Verification items for the finished model (mm, model axes). Face numbers are marked on the shaded views. A direction names the side the tool comes from. Round coordinates to 2 decimals unless told otherwise and drop trailing zeros. Loops run counter-clockwise (first coordinate to the right, second up) from the corner with the lowest first, then second, coordinate; pieces in that order, holes last. Notation, with made-up numbers: (-33, 42.5) -> (-25, 42.5) arc R19 ccw to (-25, 54.5) -> close; hole circle Ø2 at (-9.5, -22.5). An arc over 180 degrees is marked (long way). Write item = value, one per line. Start each with the question number.
```python
from build123d import *

# Parameters (mm, degrees)
F1_DEPTH = 1.27
F2_W     = 3.175
F2_H     = 3.175
F3_DEPTH = 25.4


with BuildPart() as f1:
    # F0 (on Front) → F1 (new body)
    with BuildSketch(Plane.XZ):
        with BuildLine():
            Line((2.9464038958, -0.7894865445), (0, 0))
            Line((0, 0), (3.0794409887, 0.8251337261))
            Line((3.0794409887, 0.8251337261), (2.99397894, 1.1440824339))
            Line((2.99397894, 1.1440824339), (3.3486255796, 1.4393611732))
            ThreePointArc((3.3486255796, 1.4393611732), (3.1918481536, 1.8075915845), (2.9973088366, 2.1573447134))
            Line((2.9973088366, 2.1573447134), (2.6208310146, 2.0564677851))
            Line((2.6208310146, 2.0564677851), (2.3873443555, 2.2899544442))
            Line((2.3873443555, 2.2899544442), (2.1538576963, 2.5234411034))
            Line((2.1538576963, 2.5234411034), (2.3133513259, 2.9564833127))
            ThreePointArc((2.3133513259, 2.9564833127), (1.9934628866, 3.1969914902), (1.6501103316, 3.4026169264))
            Line((1.6501103316, 3.4026169264), (1.374509438, 3.1270160328))
            Line((1.374509438, 3.1270160328), (1.0555607301, 3.2124780815))
            Line((1.0555607301, 3.2124780815), (0.7366120223, 3.2979401302))
            Line((0.7366120223, 3.2979401302), (0.6582164526, 3.7527124992))
            ThreePointArc((0.6582164526, 3.7527124992), (0.2609308491, 3.8010544711), (-0.1392339042, 3.807455045))
            Line((-0.1392339042, 3.807455045), (-0.2401108325, 3.430977223))
            Line((-0.2401108325, 3.430977223), (-0.5590595404, 3.3455151743))
            Line((-0.5590595404, 3.3455151743), (-0.8780082482, 3.2600531257))
            Line((-0.8780082482, 3.2600531257), (-1.1732869876, 3.6146997653))
            ThreePointArc((-1.1732869876, 3.6146997653), (-1.5415173988, 3.4579223392), (-1.8912705277, 3.2633830223))
            Line((-1.8912705277, 3.2633830223), (-1.7903935994, 2.8869052003))
            Line((-1.7903935994, 2.8869052003), (-2.0238802585, 2.6534185411))
            Line((-2.0238802585, 2.6534185411), (-2.2573669177, 2.419931882))
            Line((-2.2573669177, 2.419931882), (-2.690409127, 2.5794255116))
            ThreePointArc((-2.690409127, 2.5794255116), (-2.9309173045, 2.2595370723), (-3.1365427408, 1.9161845173))
            Line((-3.1365427408, 1.9161845173), (-2.8609418471, 1.6405836237))
            Line((-2.8609418471, 1.6405836237), (-2.9464038958, 1.3216349158))
            Line((-2.9464038958, 1.3216349158), (-3.0318659445, 1.002686208))
            Line((-3.0318659445, 1.002686208), (-3.4866383135, 0.9242906383))
            ThreePointArc((-3.4866383135, 0.9242906383), (-3.5349802854, 0.5270050347), (-3.5413808594, 0.1268402815))
            Line((-3.5413808594, 0.1268402815), (-3.1649030374, 0.0259633531))
            Line((-3.1649030374, 0.0259633531), (-3.0794409887, -0.2929853547))
            Line((-3.0794409887, -0.2929853547), (-2.99397894, -0.6119340625))
            Line((-2.99397894, -0.6119340625), (-3.3486255796, -0.9072128019))
            ThreePointArc((-3.3486255796, -0.9072128019), (-3.1918481536, -1.2754432131), (-2.9973088366, -1.6251963421))
            Line((-2.9973088366, -1.6251963421), (-2.6208310146, -1.5243194137))
            Line((-2.6208310146, -1.5243194137), (-2.3873443555, -1.7578060728))
            Line((-2.3873443555, -1.7578060728), (-2.1538576963, -1.991292732))
            Line((-2.1538576963, -1.991292732), (-2.3133513259, -2.4243349413))
            ThreePointArc((-2.3133513259, -2.4243349413), (-1.9934628866, -2.6648431188), (-1.6501103316, -2.8704685551))
            Line((-1.6501103316, -2.8704685551), (-1.374509438, -2.5948676615))
            Line((-1.374509438, -2.5948676615), (-1.0555607301, -2.6803297101))
            Line((-1.0555607301, -2.6803297101), (-0.7366120223, -2.7657917588))
            Line((-0.7366120223, -2.7657917588), (-0.6582164526, -3.2205641278))
            ThreePointArc((-0.6582164526, -3.2205641278), (-0.2609308491, -3.2689060997), (0.1392339042, -3.2753066737))
            Line((0.1392339042, -3.2753066737), (0.2401108325, -2.8988288517))
            Line((0.2401108325, -2.8988288517), (0.5590595404, -2.813366803))
            Line((0.5590595404, -2.813366803), (0.8780082482, -2.7279047543))
            Line((0.8780082482, -2.7279047543), (1.1732869876, -3.0825513939))
            ThreePointArc((1.1732869876, -3.0825513939), (1.5415173988, -2.9257739679), (1.8912705277, -2.7312346509))
            Line((1.8912705277, -2.7312346509), (1.7903935994, -2.3547568289))
            Line((1.7903935994, -2.3547568289), (2.0238802585, -2.1212701698))
            Line((2.0238802585, -2.1212701698), (2.2573669177, -1.8877835106))
            Line((2.2573669177, -1.8877835106), (2.690409127, -2.0472771403))
            ThreePointArc((2.690409127, -2.0472771403), (2.9309173045, -1.7273887009), (3.1365427408, -1.3840361459))
            Line((3.1365427408, -1.3840361459), (2.8609418471, -1.1084352523))
            Line((2.8609418471, -1.1084352523), (2.9464038958, -0.7894865445))
        make_face()
        with BuildLine():
            ThreePointArc((3.4866383135, -0.392142267), (3.4939098929, -0.3492466485), (3.5006911676, -0.3062707917))
            Line((3.5006911676, -0.3062707917), (0, 0))
            Line((0, 0), (2.9464038958, -0.7894865445))
            Line((2.9464038958, -0.7894865445), (3.0318659445, -0.4705378366))
            Line((3.0318659445, -0.4705378366), (3.4866383135, -0.392142267))
        make_face()
        with BuildLine():
            ThreePointArc((3.5439258143, 0.2660741857), (3.5438624188, 0.2880530324), (3.5436722344, 0.3100311478))
            Line((3.5436722344, 0.3100311478), (0, 0))
            Line((0, 0), (3.5006911676, -0.3062707917))
            ThreePointArc((3.5006911676, -0.3062707917), (3.5331017773, -0.0209136223), (3.5439258143, 0.2660741857))
        make_face()
        with BuildLine():
            Line((0, 0), (3.5436722344, 0.3100311478))
            ThreePointArc((3.5436722344, 0.3100311478), (3.5428244693, 0.3576767837), (3.5413808594, 0.4053080898))
            Line((3.5413808594, 0.4053080898), (3.1649030374, 0.5061850182))
            Line((3.1649030374, 0.5061850182), (3.0794409887, 0.8251337261))
            Line((3.0794409887, 0.8251337261), (0, 0))
        make_face()
    extrude(amount=F1_DEPTH)

    # F2 (on face) → F3 (cut)
    with BuildSketch(Plane.XZ.offset(1.27)):
        with Locations((0, 0.2660741857)):
            Rectangle(F2_W, F2_H)
    extrude(amount=-F3_DEPTH, mode=Mode.SUBTRACT)


solid = f1.part
```
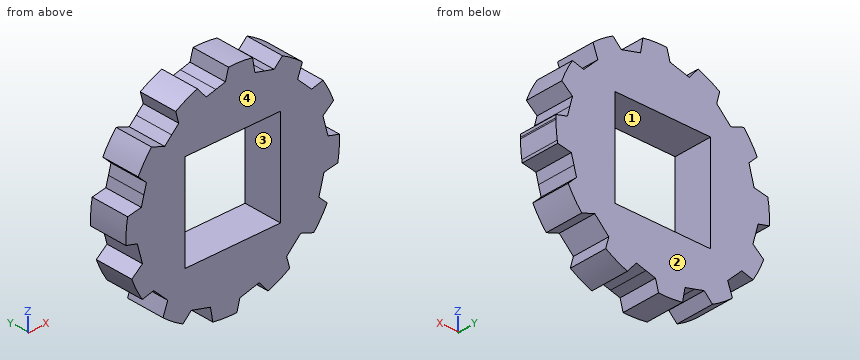
(1) Draft check along Z on the marked faces 3 and 4. Enter one of: +Z half, -Z half, draft (parallel to the pull), parting line (faces both ways), or undercut.
(2) Section check C-C on x = -2.5. Enter the section's corners in (y, z), then the cut area to 3 significant figures.
(3) Section check A-A on z = 1.75. Enter the section's corners in (x, y), then the cut area to 3 significant figures.
(4) Section check B-B on x = 1.5. Enter the section's corners in (y, z).
(5) Scan lines: line 1 (X direction, y = -0.6, z = -0.25); line 2 (X direction, y = -0.3, z = 1.75); line 3 (Z direction, x = -1, y = -1.1). Record each from-to range of solid material in increasing order. Write a range as [from, to].
(6) Access from +Z, -Z, +X, -X, +Y, -Y to the whole of each face (thin tool, end or side, straight path). Record for the marked faces 1 and 2.
(7) Section check D-D on z = -1.75. Enter the section's corners in (x, y), then the cut area to 3 significant figures.
(8) Depth check by flat-ended pin: pin 1 Ø0.6 at (y, z) = (-0.5, 0) entering from -X. Enter the tip coordinate at first touch or a pass-through.
Computed values:
q1.face_3 = undercut
q1.face_4 = draft
q2.outline = (-1.27, -1.65) -> (0, -1.65) -> (0, 2.51) -> (-1.27, 2.51) -> close
q2.area = 5.28 mm²
q3.outline = (-2.97, -1.27) -> (-1.59, -1.27) -> (-1.59, 0) -> (-2.97, 0) -> close; (1.59, -1.27) -> (3.22, -1.27) -> (3.22, 0) -> (1.59, 0) -> close
q3.area = 3.83 mm²
q4.outline = (-1.27, -2.95) -> (0, -2.95) -> (0, -1.32) -> (-1.27, -1.32) -> close; (-1.27, 1.85) -> (0, 1.85) -> (0, 3.25) -> (-1.27, 3.25) -> close
q5.line_1 = [-3.09, -1.59], [1.59, 3.51]
q5.line_2 = [-2.97, -1.59], [1.59, 3.22]
q5.line_3 = [-2.7, -1.32], [1.85, 3.41]
q6.face_1 = +Y, -Y
q6.face_2 = +Z, -Z, +X, -X, +Y
q7.outline = (-2.4, -1.27) -> (2.92, -1.27) -> (2.92, 0) -> (-2.4, 0) -> close
q7.area = 6.74 mm²
q8.pin_1 = -3.54
